```python
from build123d import *

# Parameters (mm, degrees)
SKETCH_R           = 9
SKETCH_R_2         = 3.15
PAD_DEPTH          = 15
SKETCH001_R        = 9
PAD001_DEPTH       = 12
FILLET_R           = 3
SKETCH002_R        = 1
POCKET_DEPTH       = 15
POLARPATTERN_COUNT = 10
SKETCH003_W        = 7.258159
SKETCH003_H        = 2.087937
PAD002_DEPTH       = 10


with BuildPart() as part:
    # Sketch → Pad (new body)
    with BuildSketch(Plane.XY):
        Circle(SKETCH_R)
        Circle(SKETCH_R_2, mode=Mode.SUBTRACT)
    extrude(amount=PAD_DEPTH)

    # Sketch001 (on Face4 of Pad) → Pad001 (join)
    with BuildSketch(Plane.XY.offset(15)):
        Circle(SKETCH001_R)
    extrude(amount=-PAD001_DEPTH)

    # Fillet
    fillet_edges = [part.edges().sort_by_distance(p)[0] for p in [
        (-9, 0, 15),
    ]]
    fillet(fillet_edges, radius=FILLET_R)

    # Sketch002 (on Face6 of Fillet) → Pocket (cut)
    with BuildSketch(Plane.XY.offset(15)):
        with Locations((9.3, 0)):
            Circle(SKETCH002_R)
    pocket = extrude(amount=-POCKET_DEPTH, mode=Mode.SUBTRACT)

    # PolarPattern: Pocket ×10 about axis
    polarpattern_axis = Axis((0, 0, 0), (0, 0, 1))
    for i in range(1, POLARPATTERN_COUNT):
        add(pocket.rotate(polarpattern_axis, i * 360 / POLARPATTERN_COUNT), mode=Mode.SUBTRACT)

    # Sketch003 (on Face8 of PolarPattern) → Pad002 (join)
    with BuildSketch(Plane(origin=(0, 0, 0), x_dir=(1, 0, 0), z_dir=(0, 0, -1))):
        with Locations((0.174419, -2.743968)):
            Rectangle(SKETCH003_W, SKETCH003_H)
    extrude(amount=-PAD002_DEPTH)


solid = part.part
```
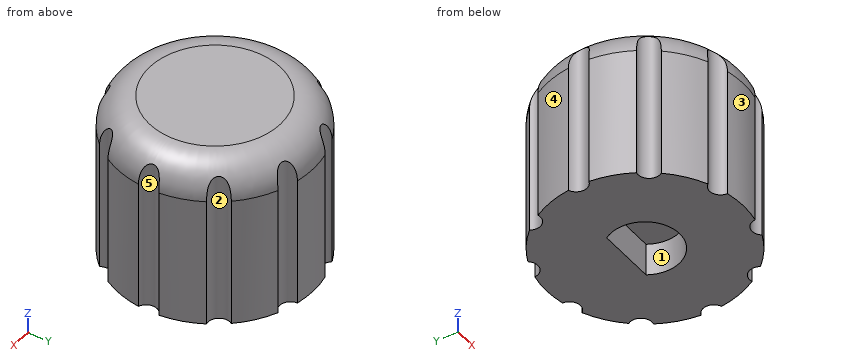
CAD build for the part. Positions are in the model's coordinates, mm. Face numbers are marked on the shaded views. A direction names the side the tool comes from. Round coordinates to 2 decimals unless told otherwise and drop trailing zeros. Loops run counter-clockwise (first coordinate to the right, second up) from the corner with the lowest first, then second, coordinate; pieces in that order, holes last. Notation, with made-up numbers: (26.5, 9.25) - (72.5, 9.25) arc R26 ccw to (72.5, 27.25) - close; hole circle Ø8 at (-9.75, 4.25). An arc over 180 degrees is marked (long way). Return JSON: item names as keys, results as strings. Group by question number.
Q1. Band-saw the part on C-C on z = 10.75. Give the cut face in (x, y).
Q2. Tool access for the marked faces 1 and 2: list every direction of +Z, -Z, +X, -X, +Y, -Y with a clear straight run to the whole face (end or side of a thin tool).
Q3. Two-plate mould, pull along Y, no slides. Class the marked faces 3, 4 and 5: +Y half, -Y half, draft (parallel to the pull), parting line (faces both ways), or undercut.
Q4. Flat gauge pins, fed straight in: pin 1 Ø2 at (y, z) = (-5, 4) entering from -X; pin 2 Ø4 at (x, z) = (5, 5.5) entering from +Y; pin 3 Ø6 at (y, z) = (-6, 6.5) entering from -X. Where does each tip first touch, or does it go through?
Q5. Drill centre lines: line 1 along Y through (x, z) = (0, 2.1); line 2 along X through (y, z) = (0, 2.3); line 3 along X through (y, z) = (5.5, 12.75). Where is each one in solid material? Low to high. Write a range as [from, to].
Q6. Band-saw the part on A-A on y = 0. Give the cut face in (x, z).
Q7. Band-saw the part on B-B on x = 0. Give the cut face in (y, z), plus the area to 3 significant figures.
Solutions:
{
 "1": {"outline": "(-8.95, -0.94) arc R9 ccw to (-7.79, -4.5) arc R1 cw to (-6.69, -6.02) arc R9 ccw to (-3.66, -8.22) arc R1 cw to (-1.87, -8.8) arc R9 ccw to (1.87, -8.8) arc R1 cw to (3.66, -8.22) arc R9 ccw to (6.69, -6.02) arc R1 cw to (7.79, -4.5) arc R9 ccw to (8.95, -0.94) arc R1 cw to (8.95, 0.94) arc R9 ccw to (7.79, 4.5) arc R1 cw to (6.69, 6.02) arc R9 ccw to (3.66, 8.22) arc R1 cw to (1.87, 8.8) arc R9 ccw to (-1.87, 8.8) arc R1 cw to (-3.66, 8.22) arc R9 ccw to (-6.69, 6.02) arc R1 cw to (-7.79, 4.5) arc R9 ccw to (-8.95, 0.94) arc R1 cw to start"},
 "2": {"face 1": "-Z", "face 2": "+Z, -Z"},
 "3": {"face 3": "-Y half", "face 4": "+Y half", "face 5": "undercut"},
 "4": {"pin 1": "stops at x = -8.06", "pin 2": "stops at y = 8.22", "pin 3": "stops at x = -8.49"},
 "5": {"line 1": "y = [-9, -3.15], [1.7, 9]", "line 2": "x = [-8.3, -3.15], [3.15, 8.3]", "line 3": "x = [-6.52, 6.52]"},
 "6": {"outline": "(-8.3, 0) - (-3.15, 0) - (-3.15, 3) - (3.15, 3) - (3.15, 0) - (8.3, 0) - (8.3, 13.93) arc R3 ccw to (6, 15) - (-6, 15) arc R3 ccw to (-8.3, 13.93) - close"},
 "7": {"outline": "(-9, 0) - (-3.15, 0) - (-3.15, 3) - (1.7, 3) - (1.7, 0) - (9, 0) - (9, 12) arc R3 ccw to (6, 15) - (-6, 15) arc R3 ccw to (-9, 12) - close", "area": "252 mm^2"}
}
